Geometry: final body of the model. Coordinates: model frame, mm. A direction names the side the tool comes from. Coordinates: 2 decimals unless noted, no trailing zeros. Loops run counter-clockwise (first coordinate to the right, second up) from the corner with the lowest first, then second, coordinate; pieces in that order, holes last. Notation, with made-up numbers: M 79.25,-34 L 86.25,-34 A20 cw 86.25,-18 Z; hole C -13,49.5 d7. An arc over 180 degrees is marked long. Write each question's results on one line, items separated by ' | '. Start each with the question number.
from build123d import *

# Parameters (mm, degrees)
SKETCH1_W                       = 152.4
SKETCH1_H                       = 76.2
SKETCH1_R                       = 3.854557775
BOSS_EXTRUDE1_DEPTH             = 19.05
F_1_4_0_25_DIAMETER_HOLE2_D     = 6.35
F_1_4_0_25_DIAMETER_HOLE2_DEPTH = 12.7
F_1_4_0_25_DIAMETER_HOLE2_TIP   = 1.907732465
SKETCH2_R                       = 4.7625
CUT_EXTRUDE1_DEPTH              = 6.35


with BuildPart() as part:
    # Sketch1 → Boss-Extrude1 (new body)
    with BuildSketch(Plane(origin=(0, 0, 0), x_dir=(0, 0, -1), z_dir=(1, 0, 0))):
        Rectangle(SKETCH1_W, SKETCH1_H)
        with Locations(Location((-38.1, 0, 0), (0, 0, 180))):
            Circle(SKETCH1_R, mode=Mode.SUBTRACT)
        with Locations(Location((-14.836022013, -7.860160654, 0), (0, 0, 180))):
            Circle(SKETCH1_R, mode=Mode.SUBTRACT)
        with Locations(Location((18.457733582, 1.096077429, 0), (0, 0, 180))):
            Circle(SKETCH1_R, mode=Mode.SUBTRACT)
        with Locations(Location((51.143457994, -9.873506971, 0), (0, 0, 180))):
            Circle(SKETCH1_R, mode=Mode.SUBTRACT)
    extrude(amount=BOSS_EXTRUDE1_DEPTH)

    # 1_4 _0.25_ Diameter Hole2
    with Locations(Plane.XZ.offset(38.1)):
        with Locations((9.525, 57.15), (9.525, -63.5), (9.525, 0)):
            Hole(F_1_4_0_25_DIAMETER_HOLE2_D / 2, depth=F_1_4_0_25_DIAMETER_HOLE2_DEPTH)
            with Locations((0, 0, -(F_1_4_0_25_DIAMETER_HOLE2_DEPTH + F_1_4_0_25_DIAMETER_HOLE2_TIP / 2))):  # 118° drill point
                Cone(0, F_1_4_0_25_DIAMETER_HOLE2_D / 2, F_1_4_0_25_DIAMETER_HOLE2_TIP, mode=Mode.SUBTRACT)

    # Sketch2 → Cut-Extrude1 (cut)
    with BuildSketch(Plane.ZY):
        with Locations((38.1, 0)):
            Circle(SKETCH2_R)
        with Locations((14.836022013, -7.860160654)):
            Circle(SKETCH2_R)
        with Locations((-18.457733582, 1.096077429)):
            Circle(SKETCH2_R)
        with Locations((-51.143457994, -9.873506971)):
            Circle(SKETCH2_R)
    extrude(amount=-CUT_EXTRUDE1_DEPTH, mode=Mode.SUBTRACT)


solid = part.part
Item 1: Section C-C, the plane x = 11.25. Count the separate pieces of the cut face and the enclosed holes in it, plus the area to 3 significant figures.
Item 2: Set-up query: faces 4 (the cylindrical face through (10.21, -31.66, 54.05)), 5 (the cylindrical face through (12.61, -0.06, -14.78)), 6 (the cylindrical face through (3.13, -7.65, 10.08)). Return all of +Z, -Z, +X, -X, +Y, -Y with unobstructed straight access to the full face (end or side cutting, diameter ignored); none if empty.
Item 3: Contact query for flat-ended pins moving along their axis: P1, Ø3, axis at y = -1, z = 36.5, coming from the -X side; P2, Ø5, axis at y = 1, z = -20, coming from the -X side. Output: stop coordinate, or through.
Item 4: Ray query, L1, parallel to X at y = -33.25, z = 0; L2, parallel to Z at x = 9.5, y = -8; L3, parallel to Y at x = 4.5, z = -48. Return the intervals inside material, ascending. Write a range as [from, to].
Item 5: Section B-B, the plane x = 1.5. Return loops of the section in (y, z) (1 decimal), plus the area to 3 significant figures.
Item 6: Section A-A, the plane z = 38.1. Return loops of the section in (x, y), plus the area to 3 significant figures.
Item 7: Pull-direction query (X, two-part tool) for faces 1 (the cylindrical face through (12.61, -9.02, 18.51)), 2 (the flat face through (19.05, 1, 1)), 3 (the conical face through (10.051, -23.824, 0.166)); classes: released by +X, released by -X, zero draft, split by the parting line, or undercut.
Solutions:
1) separate pieces: 1 | enclosed holes: 4 | area: 11,200 mm²
2) face 4: -Y | face 5: +X, -X | face 6: -X
3) P1: passes through | P2: stops at x = 6.35
4) L1: x = [0, 6.35], [12.7, 19.05] | L2: z = [-76.2, -54.51], [-47.77, 10.98], [18.69, 76.2] | L3: y = [-38.1, -13.45], [-6.3, 38.1]
5) outline: M -38.1,-76.2 L 38.1,-76.2 L 38.1,76.2 L -38.1,76.2 Z; hole C -9.9,-51.1 d9.5; hole C -7.9,14.8 d9.5; hole C 0,38.1 d9.5; hole C 1.1,-18.5 d9.5 | area: 11,300 mm²
6) outline: M 0,-38.1 L 19.05,-38.1 L 19.05,-3.85 L 6.35,-3.85 L 6.35,-4.76 L 0,-4.76 Z; M 0,4.76 L 6.35,4.76 L 6.35,3.85 L 19.05,3.85 L 19.05,38.1 L 0,38.1 Z | area: 1,290 mm²
7) face 1: zero draft | face 2: released by +X | face 3: undercut
